Geometry: final body of the model. Coordinates: model frame, mm. A direction names the side the tool comes from. Round coordinates to 2 decimals unless told otherwise and drop trailing zeros. Write each loop counter-clockwise with the first axis right and the second up, starting at its lowest first coordinate (ties: lowest second). Pieces come first, ordered by that corner, then holes. Notation, with made-up numbers: M 43,-4 L 93,-4 A17 cw 93,4 Z; hole C 14,25 d7. An arc over 180 degrees is marked long. Answer as CSV lines item,"result". Start each with the question number.
Q1. Section query A-A on y = 1.25. Give the number of separate pieces and of enclosed holes in the cut face, and give its area (3 significant figures).
Q2. Ray query, probe 1 along Z at (x, y) = (147.5, 2); probe 2 along Z at (x, y) = (-27, 2.25); probe 3 along X at (y, z) = (2.45, 163.5). Return the intervals inside material, ascending.
Q3. First-contact query: pin 1 (1.5 mm diameter, centred on x = -117.5, y = 1.5, fed in from -Z); pin 2 (1.1 mm diameter, centred on y = 3.5, z = -168, fed in from -X); pin 3 (0.8 mm diameter, centred on y = 2.5, z = -168, fed in from +X). Flat tips, straight axial feed; report the tip coordinate or a pass-through.
Q4. Reachability of faces 4 (the flat face through (136, 3, 162)), 5 (the flat face through (-2, 0, 1)), 6 (the cylindrical face through (-34.51, 3.22, -156.78)) from +Z, -Z, +X, -X, +Y, -Y: full face, straight path, thin tool, end or side. Return the list, or none.
Q5. Mould query, pull axis X, two halves, no side actions, for faces 1 (the cylindrical face through (34.51, 3.22, -156.78)), 2 (the conical face through (0.3, 3.92, -168.75)), 3 (the flat face through (-2, 6.35, 1)). Classes: pulls with the +X half, pulls with the -X half, needs draft (parallel to the pull), parting line crosses it, or undercut.
Q6. Section query B-B on x = -77. Output: boundary loops of the cut face in (y, z).
```python
from build123d import *

# Parameters (mm, degrees)
BOSS_EXTRUDE1_DEPTH                             = 6.35
CSK_FOR_M4_FLAT_HEAD_MACHINE_SCREW1_D           = 4.3
CSK_FOR_M4_FLAT_HEAD_MACHINE_SCREW1_CSINK_D     = 9.4
CSK_FOR_M4_FLAT_HEAD_MACHINE_SCREW1_CSINK_ANGLE = 90
CHAMFER1_SIZE                                   = 16
SKETCH6_W                                       = 10
SKETCH6_H                                       = 6
BOSS_EXTRUDE2_DEPTH                             = 6.35
FILLET5_R                                       = 8
M3X0_5_TAPPED_HOLE1_D                           = 2.5
FILLET6_START                                   = -1
FILLET6_DEPTH                                   = 8
SKETCH18_W                                      = 25
SKETCH18_H                                      = 19
BOSS_EXTRUDE4_DEPTH                             = 6.35
FILLET11_R                                      = 15
FILLET12_R                                      = 3
TAP_DRILL_FOR_M3X0_5_TAP2_D                     = 2.5


with BuildPart() as part:
    # Sketch1 → Boss-Extrude1 (new body)
    with BuildSketch(Plane(origin=(0, 0, 0), x_dir=(1, 0, 0), z_dir=(0, 1, 0))):
        Polygon((-5, 171.5), (5, 171.5), (5, 152.5), (152.5, 152.5), (152.5, -168.5), (142.5, -168.5), (142.5, -152.5), (-142.5, -152.5), (-142.5, -168.5), (-152.5, -168.5), (-152.5, 152.5), (-5, 152.5), align=None)
    extrude(amount=BOSS_EXTRUDE1_DEPTH)

    # CSK for M4 Flat Head Machine Screw1 (through all)
    with Locations(Plane(origin=(0, 6.35, 0), x_dir=(1, 0, 0), z_dir=(0, 1, 0))):
        with Locations((0, 166.5), (-147.5, -163.5), (147.5, -163.5)):
            CounterSinkHole(CSK_FOR_M4_FLAT_HEAD_MACHINE_SCREW1_D / 2, CSK_FOR_M4_FLAT_HEAD_MACHINE_SCREW1_CSINK_D / 2, counter_sink_angle=CSK_FOR_M4_FLAT_HEAD_MACHINE_SCREW1_CSINK_ANGLE)

    # Chamfer1
    chamfer1_edges = [part.edges().sort_by_distance(p)[0] for p in [
        (142.5, 3.175, 152.5),
        (-142.5, 3.175, 152.5),
    ]]
    chamfer(chamfer1_edges, length=CHAMFER1_SIZE - 0.0001)  # a hair under: the kernel refuses the full size

    # Sketch6 → Boss-Extrude2 (add)
    with BuildSketch(Plane(origin=(0, 6.35, 0), x_dir=(1, 0, 0), z_dir=(0, 1, 0))):
        with Locations((-147.5, 155.5)):
            Rectangle(SKETCH6_W, SKETCH6_H)
        with Locations((147.5, 155.5)):
            Rectangle(SKETCH6_W, SKETCH6_H)
    extrude(amount=-BOSS_EXTRUDE2_DEPTH)

    # Fillet5
    # the kernel refuses this fillet: 8 mm, written as the material it adds along each edge
    with BuildSketch(Plane(origin=(142.5, 6.35, -152.5), x_dir=(0, 0, -1), z_dir=(0, -1, 0))) as fillet5_piece_1:
        with BuildLine():
            CenterArc((8, -7.745966692), FILLET5_R, 104.477512186, 75.522487814)
            Line((0, -7.745966692), (-0.16, -7.745966692))
            Line((-0.16, -7.745966692), (-0.16, 0))
            Line((-0.16, 0), (0, 0.16))
            ThreePointArc((0, 0.16), (3, 0.16), (5.96, 0.154919334))
            Line((5.96, 0.154919334), (6, 0))
        make_face()
    extrude(amount=6.35)
    with BuildSketch(Plane(origin=(-142.5, 6.35, -152.5), x_dir=(1, 0, 0), z_dir=(0, -1, 0))) as fillet5_piece_2:
        with BuildLine():
            CenterArc((7.745966692, -8), FILLET5_R, 90, 75.522487814)
            Line((0, -6), (-0.154919334, -5.96))
            ThreePointArc((-0.154919334, -5.96), (-0.16, -3), (-0.16, 0))
            Line((-0.16, 0), (0, 0.16))
            Line((0, 0.16), (7.745966692, 0.16))
            Line((7.745966692, 0.16), (7.745966692, 0))
        make_face()
    extrude(amount=6.35)

    # M3x0.5 Tapped Hole1 (through all)
    with Locations(Plane(origin=(0, 6.35, 0), x_dir=(1, 0, 0), z_dir=(0, 1, 0))):
        with Locations((-147.5, 154), (147.5, 154), (137.107695155, -157.5), (-137.107695155, -157.5), (0, 155.5)):
            Hole(M3X0_5_TAPPED_HOLE1_D / 2)

    # Fillet6: read off the stored shape, not the designer's step
    # Fillet6 outline → Fillet6 (cut)
    with BuildSketch(Plane(origin=(0, 0, 0), x_dir=(1, 0, 0), z_dir=(0, 1, 0)).offset(FILLET6_START)):
        with BuildLine():
            ThreePointArc((152.5, -163.5), (151.035533906, -167.035533906), (147.5, -168.5))
            Line((147.5, -168.5), (152.5, -168.5))
            Line((152.5, -168.5), (152.5, -163.5))
        make_face()
        with BuildLine():
            ThreePointArc((144.571067812, -168.5), (142.65765065, -168.119397663), (141.035533906, -167.035533906))
            Line((141.035533906, -167.035533906), (142.5, -168.5))
            Line((142.5, -168.5), (144.571067812, -168.5))
        make_face()
        with BuildLine():
            ThreePointArc((-141.035533906, -167.035533906), (-142.65765065, -168.119397663), (-144.571067812, -168.5))
            Line((-144.571067812, -168.5), (-142.5, -168.5))
            Line((-142.5, -168.5), (-141.035533906, -167.035533906))
        make_face()
        with BuildLine():
            Line((-152.5, -168.5), (-147.5, -168.5))
            ThreePointArc((-147.5, -168.5), (-151.035533906, -167.035533906), (-152.5, -163.5))
            Line((-152.5, -163.5), (-152.5, -168.5))
        make_face()
    extrude(amount=FILLET6_DEPTH, mode=Mode.SUBTRACT)

    # Sketch18 → Boss-Extrude4 (add)
    with BuildSketch(Plane.XZ):
        with Locations((17.5, -162)):
            Rectangle(SKETCH18_W, SKETCH18_H)
        with Locations((-17.5, -162)):
            Rectangle(SKETCH18_W, SKETCH18_H)
    extrude(amount=-BOSS_EXTRUDE4_DEPTH)

    # Fillet11
    fillet11_edges = [part.edges().sort_by_distance(p)[0] for p in [
        (30, 3.175, -152.5),
        (-30, 3.175, -152.5),
        (-126.5001, 3.175, 152.5),
        (126.5001, 3.175, 152.5),
    ]]
    fillet(fillet11_edges, radius=FILLET11_R)

    # Fillet12
    fillet12_edges = [part.edges().sort_by_distance(p)[0] for p in [
        (30, 3.175, -171.5),
        (-30, 3.175, -171.5),
        (-142.5, 3.175, -158.5),
        (-152.5, 3.175, -158.5),
        (142.5, 3.175, -158.5),
        (152.5, 3.175, -158.5),
    ]]
    fillet(fillet12_edges, radius=FILLET12_R)

    # Tap Drill for M3x0.5 Tap2 (through all)
    with Locations(Plane(origin=(0, 6.35, 0), x_dir=(1, 0, 0), z_dir=(0, 1, 0))):
        with Locations((27, 154.5), (-27, 168.5), (-27, 158.5)):
            Hole(TAP_DRILL_FOR_M3X0_5_TAP2_D / 2)


solid = part.part
```
Entries:
1,separate pieces,"1"
1,enclosed holes,"11"
1,area,"94,900 mm^2"
2,probe 1,"z = -158.5 to -155.25, -152.75 to 161.35, 165.65 to 168.5"
2,probe 2,"z = -171.5 to -169.75, -167.25 to -159.75, -157.25 to 152.5"
2,probe 3,"x = -152.5 to -149.65, -145.35 to -137.5, 137.5 to 145.35, 149.65 to 152.5"
3,pin 1,"stops at z = -152.5"
3,pin 2,"stops at x = -30"
3,pin 3,"stops at x = 30"
4,face 4,"+Z, +Y, -Y"
4,face 5,"+Z, -Z, +X, -X, -Y"
4,face 6,"-Z, +Y, -Y"
5,face 1,"undercut"
5,face 2,"undercut"
5,face 3,"needs draft"
6,outline,"M 0,-152.5 L 6.35,-152.5 L 6.35,152.5 L 0,152.5 Z"
